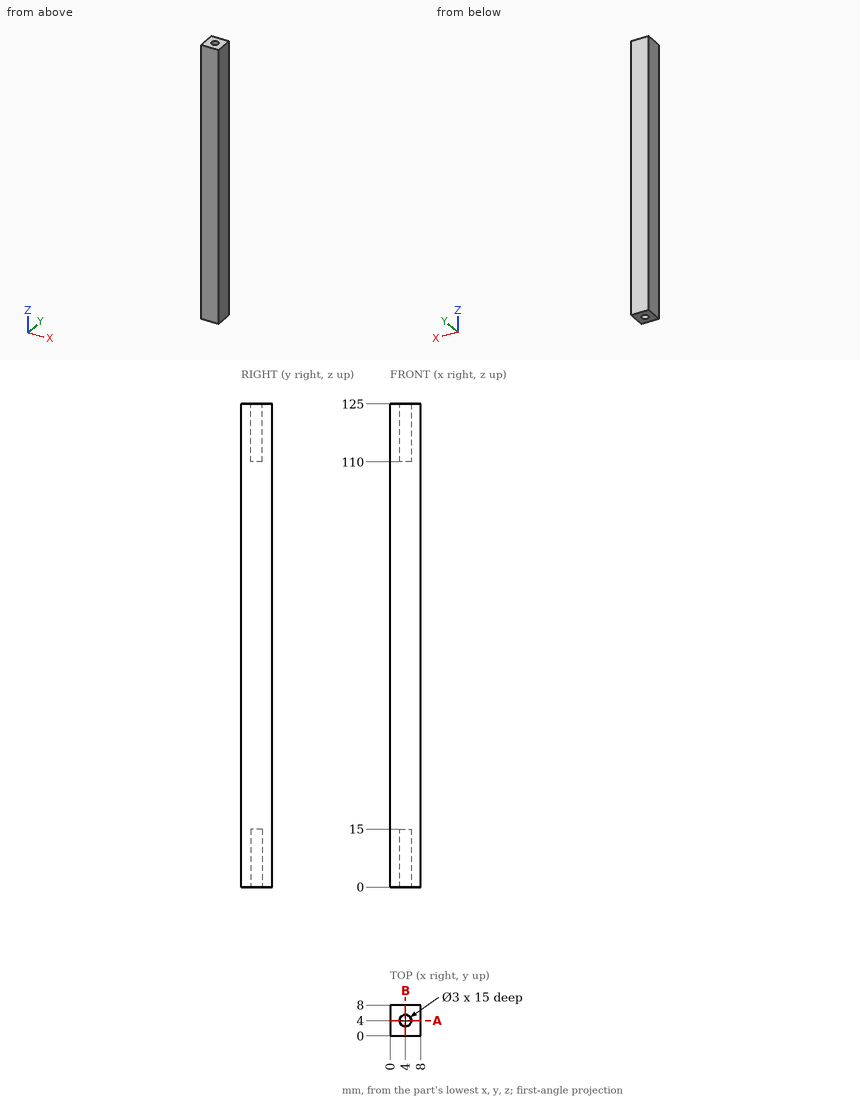
Source: three-view drawing plus pictorial views. Frame: mm from the lowest corner of the part. Round coordinates to 2 decimals unless told otherwise and drop trailing zeros. Loops run counter-clockwise (first coordinate to the right, second up) from the corner with the lowest first, then second, coordinate; pieces in that order, holes last.
1. Ray query, L1, parallel to Y at x = 4, z = 117.5; L2, parallel to X at y = 5, z = 111.5; L3, parallel to Z at x = 3.25, y = 5.25. Return the intervals inside material, ascending.
2. Section query A-A on y = 4. Output: boundary loops of the cut face in (x, z), and give its area (3 significant figures).
3. Contact query for flat-ended pins moving along their axis: pin 1 (2 mm diameter, centred on x = 3.5, y = 1, fed in from -Z); pin 2 (2.5 mm diameter, centred on x = 4, y = 4, fed in from +Z). Output: stop coordinate, or through.
Answers below:
1. L1: y = 0 to 2.5, 5.5 to 8
1. L2: x = 0 to 2.88, 5.12 to 8
1. L3: z = 15 to 110
2. outline: (0, 0) - (2.5, 0) - (2.5, 15) - (5.5, 15) - (5.5, 0) - (8, 0) - (8, 125) - (5.5, 125) - (5.5, 110) - (2.5, 110) - (2.5, 125) - (0, 125) - close
2. area: 910 mm2
3. pin 1: stops at z = 0
3. pin 2: stops at z = 110
